Part model, mm, in its own coordinate system. Coordinates: 2 decimals unless noted, no trailing zeros. Order: outer loops, then holes, each group sorted by start corner. A loop starts at its lowest first (then second) coordinate and runs counter-clockwise, first axis right, second up. Notation, with made-up numbers: (70, 6.5) - (84, 6.5) arc R34 ccw to (84, 43.5) - close; hole circle Ø1 at (-6.75, 24.5). An arc over 180 degrees is marked (long way). Use a Markdown table: item, result. Add a question column.
1) Drop flat-ended pins along their axis: P1, Ø1, axis at x = 90, z = -2.5, coming from the -Y side; P2, Ø10, axis at x = -65.89, z = 0, coming from the +Y side; P3, Ø4, axis at y = -43.5, z = -4, coming from the -X side. Give the stop position or say it passes through.
2) Wall check: L1, parallel to X at y = -31, z = 2.25 (3 decimals); L2, parallel to X at y = 2, z = 1.25 (3 decimals); L3, parallel to X at y = -20, z = 1.75 (3 decimals). Give the ranges that are in metal, low to high. Write a range as [from, to].
3) Saw through at A-A on x = 45.5. List the corners of the cut face in (y, z) (3 decimals).
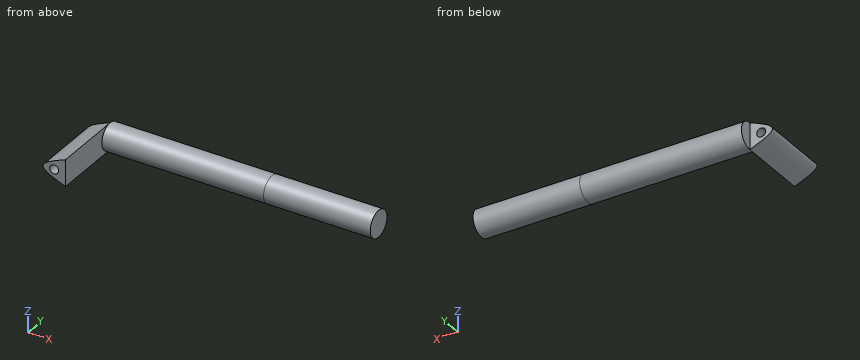
```python
from build123d import *

# Parameters (mm, degrees)
F0_R     = 9.525
F1_DEPTH = 57.785
F2_R     = 3.175
F3_DEPTH = 50.8
F4_R     = 9.525
F5_DEPTH = 76.2


with BuildPart() as f1:
    # F0 (on Right) → F1 (new body, symmetric)
    with BuildSketch(Plane.YZ):
        Circle(F0_R)
    extrude(amount=F1_DEPTH, both=True)

    # F2 (on Front) → F3 (join)
    with BuildSketch(Plane.XZ):
        with BuildLine():
            Line((-57.785, -9.525), (-57.785, 0))
            Line((-57.785, 0), (-57.785, 9.525))
            add(Edge.make_bspline(
                [(-57.785, -9.525), (-65.827919, -6.35), (-81.913757, 0), (-65.827919, 6.35), (-57.785, 9.525)],
                knots=[0, 0, 0, 0, 18.694379, 37.388758, 37.388758, 37.388758, 37.388758], degree=3))
        make_face()
        with Locations((-65.888949, 0)):
            Circle(F2_R, mode=Mode.SUBTRACT)
    extrude(amount=F3_DEPTH)

    # F4 (on face) → F5 (join)
    with BuildSketch(Plane.YZ.offset(57.785)):
        Circle(F4_R)
    extrude(amount=F5_DEPTH)


solid = f1.part
```
Results are:
| question | item | result |
|---|---|---|
| 1 | P1 | y = -9.31 |
| 1 | P2 | y = 0 |
| 1 | P3 | x = -72.88 |
| 2 | L1 | [-72.63, -68.129], [-63.649, -57.785] |
| 2 | L2 | [-57.785, 133.985] |
| 2 | L3 | [-73.106, -68.538], [-63.24, -57.785] |
| 3 | outline | circle Ø19.05 at (0, 0) |
